from build123d import *

# Parameters (mm, degrees)
F0_R          = 7.5
F1_DEPTH      = 2
F0_R_2        = 7.25
F2_DEPTH      = 2
F3_DEPTH      = 2
F3_DEPTH_BACK = 2


with BuildPart() as f1:
    # F0 (on Front) → F1 (new body)
    with BuildSketch(Plane.XZ):
        with BuildLine():
            Line((-8, 10), (-8, -10))
            Line((-8, -10), (0, -10))
            ThreePointArc((0, -10), (10, 0), (0, 10))
            Line((0, 10), (-8, 10))
        make_face()
        Circle(F0_R, mode=Mode.SUBTRACT)
        with BuildLine():
            Line((-10, 10), (-10, 0))
            ThreePointArc((-10, 0), (-12.928932, -7.071068), (-20, -10))
            Line((-20, -10), (-8, -10))
            Line((-8, -10), (-8, 10))
            Line((-8, 10), (-10, 10))
        make_face()
    extrude(amount=F1_DEPTH)

    # F0 (on Front) → F2 (join)
    with BuildSketch(Plane.XZ):
        with BuildLine():
            Line((-10, 10), (-10, 0))
            ThreePointArc((-10, 0), (-12.928932, -7.071068), (-20, -10))
            Line((-20, -10), (-8, -10))
            Line((-8, -10), (-8, 10))
            Line((-8, 10), (-10, 10))
        make_face()
        with BuildLine():
            ThreePointArc((-20, -10), (-12.928932, -7.071068), (-10, 0))
            Line((-10, 0), (-10, 10))
            Line((-10, 10), (-20, 10))
            ThreePointArc((-20, 10), (-30, 0), (-20, -10))
        make_face()
        with Locations((-20, 0)):
            Circle(F0_R_2, mode=Mode.SUBTRACT)
    extrude(amount=-F2_DEPTH)

    # F0 (on Front) → F3 (join, two sides)
    with BuildSketch(Plane.XZ) as f3_sk:
        with Locations((-20, 0)):
            Circle(F0_R_2)
    extrude(amount=F3_DEPTH)
    extrude(f3_sk.sketch, amount=-F3_DEPTH_BACK)


solid = f1.part
Geometry check sheet. Reference: the model listing, model coordinates, mm. A direction names the side the tool comes from. Round coordinates to 2 decimals unless told otherwise and drop trailing zeros. Write each loop counter-clockwise with the first axis right and the second up, starting at its lowest first coordinate (ties: lowest second). Pieces come first, ordered by that corner, then holes. Notation, with made-up numbers: (21, -36) - (75, -36) arc R17 ccw to (75, -9) - close; hole circle Ø8 at (-26, 63). An arc over 180 degrees is marked (long way). One line per item, written item: value.
1. Cross-section at A-A on y = -0.5. Record the boundary of the cut face in (x, z).
The answers:
outline: circle Ø14.5 at (-20, 0); (-20, -10) - (0, -10) arc R10 ccw to (0, 10) - (-10, 10) - (-10, 0) arc R10 cw to start; hole circle Ø15 at (0, 0)
2. Scan lines: L1, parallel to X at y = -0.35, z = -3; L2, parallel to X at y = -1.45, z = 2; L3, parallel to Z at x = -17, y = -0.4. Record each from-to range of solid material in increasing order.
The answers:
L1: x = -26.6 to -13.4, -10.46 to -6.87, 6.87 to 9.54
L2: x = -26.97 to -13.03, -10 to -7.23, 7.23 to 9.8
L3: z = -10 to -9.54, -6.6 to 6.6
3. Set-up check for faces 4 (the face through (-8, 1, 0)), 5 (the face through (-10, -1, 5)), 6 (the face through (-13, 0, 5)), 7 (the face through (-30, 1, 0)): record each of +Z, -Z, +X, -X, +Y, -Y from which the full face is reachable in a straight line by a thin tool's end or side.
The answers:
face 4: +Z, -Z, +X, +Y
face 5: +Z, -Y
face 6: -Y
face 7: -X, +Y, -Y
4. Mould release check, pull along Z, two halves, no side actions. Record for faces 1 (the face through (-12, 0, -10)), 2 (the face through (-12.85, -0.99, -6.99)), 3 (the face through (7, 0, 5)): released by +Z, released by -Z, zero draft, split by the parting line, or undercut.
The answers:
face 1: released by -Z
face 2: undercut
face 3: zero draft
5. Cross-section at D-D on x = -12. Record the boundary of the cut face in (y, z), and give its area (3 significant figures).
The answers:
outline: (-2, -10) - (2, -10) - (2, 10) - (0, 10) - (0, -6) - (-2, -6) - close
area: 48.0 mm^2
6. Cross-section at B-B on x = 4. Record the boundary of the cut face in (y, z), and give its area (3 significant figures).
The answers:
outline: (-2, -9.17) - (0, -9.17) - (0, -6.34) - (-2, -6.34) - close; (-2, 6.34) - (0, 6.34) - (0, 9.17) - (-2, 9.17) - close
area: 11.3 mm^2
7. Cross-section at C-C on z = -5.5. Record the boundary of the cut face in (x, y), and give its area (3 significant figures).
The answers:
outline: (-28.35, 0) - (-24.72, 0) - (-24.72, -2) - (-15.28, -2) - (-15.28, 0) - (-11.65, 0) - (-11.65, -2) - (-5.1, -2) - (-5.1, 0) - (-8, 0) - (-8, 2) - (-28.35, 2) - close; (5.1, -2) - (8.35, -2) - (8.35, 0) - (5.1, 0) - close
area: 79.2 mm^2
8. Depth check by flat-ended pin: pin 1 Ø6 at (x, z) = (1, -7.5) entering from +Y; pin 2 Ø1.6 at (y, z) = (0.5, 1.5) entering from +X. Enter the tip coordinate at first touch or a pass-through.
The answers:
pin 1: stops at y = 0
pin 2: stops at x = 9.96
